Work out the finished part from the listing and answer in its coordinate system (mm). Give positions to 0.01 mm unless a question says otherwise; leave off trailing zeros. Loops run counter-clockwise (first coordinate to the right, second up) from the corner with the lowest first, then second, coordinate; pieces in that order, holes last. Notation, with made-up numbers: (86, 45) - (96, 45) arc R15 ccw to (96, 59) - close; hole circle Ø8 at (86.25, -20.75). An arc over 180 degrees is marked (long way). One line per item, written item: value.
from build123d import *

# Parameters (mm, degrees)
F0_R     = 0.5
F1_DEPTH = 1


with BuildPart() as f1:
    # F0 (on Front) → F1 (new body)
    with BuildSketch(Plane.XZ):
        with BuildLine():
            Line((-6.060225, -1.489079), (0.180674, -1.489079))
            ThreePointArc((0.180674, -1.489079), (1.5, -0.000648), (0.181961, 1.488922))
            Line((0.181961, 1.488922), (-3.121307, 1.892615))
            ThreePointArc((-3.121307, 1.892615), (-3.748768, 2.222398), (-4, 2.88523))
            Line((-4, 2.88523), (-4, 3))
            Line((-4, 3), (-8.060225, 3))
            Line((-8.060225, 3), (-8.060225, 0.510921))
            ThreePointArc((-8.060225, 0.510921), (-7.474438, -0.903293), (-6.060225, -1.489079))
        make_face()
        Circle(F0_R, mode=Mode.SUBTRACT)
    extrude(amount=F1_DEPTH)


solid = f1.part
1. Section B-B (z = 0) is taken. Write down the section's boundary in (x, y), and give its area (3 significant figures).
Output:
outline: (-7.99, -1) - (-0.5, -1) - (-0.5, 0) - (-7.99, 0) - close; (0.5, -1) - (1.5, -1) - (1.5, 0) - (0.5, 0) - close
area: 8.49 mm²
2. Section D-D (x = -2) is taken. Write down the section's boundary in (y, z).
Output:
outline: (-1, -1.49) - (0, -1.49) - (0, 1.76) - (-1, 1.76) - close
3. The mould has two halves that part along X. Classify faces 1 (the cylindrical face through (-0.108, -0.493, -0.488)), 2 (the flat face through (-3, -0.5, -1.489)), 3 (the flat face through (-8.06, -0.5, 1.8)), 4 (the flat face through (-1.45, -0.49, 1.69)): released by +X, released by -X, zero draft, split by the parting line, or undercut.
Output:
face 1: undercut
face 2: zero draft
face 3: released by -X
face 4: released by +X
4. Section C-C (y = -0.8) is taken. Write down the section's boundary in (x, z), and give its area (3 significant figures).
Output:
outline: (-8.06, 0.51) arc R2 ccw to (-6.06, -1.49) - (0.18, -1.49) arc R1.5 ccw to (0.18, 1.49) - (-3.12, 1.89) arc R1 cw to (-4, 2.89) - (-4, 3) - (-8.06, 3) - close; hole circle Ø1 at (0, 0)
area: 33.3 mm²
5. Find the intervals of material crossed by line 1 along X through (y, z) = (-0.85, -0.15); line 2 along X through (y, z) = (-0.8, 2.85); line 3 along Z through (x, y) = (0, -0.6), in increasing order.
Output:
line 1: x = -7.95 to -0.48, 0.48 to 1.49
line 2: x = -8.06 to -4
line 3: z = -1.49 to -0.5, 0.5 to 1.51
6. Section A-A (x = 0) is taken. Write down the section's boundary in (y, z).
Output:
outline: (-1, -1.49) - (0, -1.49) - (0, -0.5) - (-1, -0.5) - close; (-1, 0.5) - (0, 0.5) - (0, 1.51) - (-1, 1.51) - close
